Read the model definition and answer for the solid it produces. Units are mm, in the model's axes. A direction names the side the tool comes from. Round coordinates to 2 decimals unless told otherwise and drop trailing zeros. Write each loop counter-clockwise with the first axis right and the second up, starting at its lowest first coordinate (ties: lowest second). Pieces come first, ordered by that corner, then holes. Notation, with made-up numbers: (29, -29) -> (52, -29) arc R18 cw to (52, -11) -> close; hole circle Ø8 at (-29, 62.5). An arc over 180 degrees is marked (long way). Return JSON: item names as keys, results as strings.
from build123d import *

# Parameters (mm, degrees)
F0_W     = 406.4
F0_H     = 508
F1_DEPTH = 3.81
F2_W     = 406.4
F2_H     = 508
F2_W_2   = 398.78
F2_H_2   = 500.38
F3_DEPTH = 38.1


with BuildPart() as f1:
    # F0 (on Front) → F1 (new body)
    with BuildSketch(Plane.XZ):
        with Locations((29.981383, 24.04566)):
            Rectangle(F0_W, F0_H)
    extrude(amount=F1_DEPTH)

    # F2 (on face) → F3 (join)
    with BuildSketch(Plane.XZ.offset(3.81)):
        with Locations((29.981383, 24.04566)):
            Rectangle(F2_W, F2_H)
        with Locations((29.981383, 24.04566)):
            Rectangle(F2_W_2, F2_H_2, mode=Mode.SUBTRACT)
    extrude(amount=F3_DEPTH)


solid = f1.part
Item 1: Section A-A (y = -33) is taken. Give the vertices of the cut face in (x, z), then the cut area to 3 significant figures.
Worked answers:
{"outline": "(-173.22, -229.95) -> (233.18, -229.95) -> (233.18, 278.05) -> (-173.22, 278.05) -> close; hole (-169.41, -226.14) -> (229.37, -226.14) -> (229.37, 274.24) -> (-169.41, 274.24) -> close", "area": "6,910 mm2"}
Item 2: Straight lines are drawn through the part: L1, parallel to X at y = -37, z = -3.5; L2, parallel to Z at x = 191, y = -40; L3, parallel to Y at x = -130, z = 112. For each, find the intervals that lie inside material, in ascending order. Write a range as [from, to].
Worked answers:
{"L1": "x = [-173.22, -169.41], [229.37, 233.18]", "L2": "z = [-229.95, -226.14], [274.24, 278.05]", "L3": "y = [-3.81, 0]"}
Item 3: A flat-ended cylindrical pin translates along its axis: pin 1 (3 mm diameter, centred on x = 139.5, z = -75.5, fed in from -Y). Find the tip coordinate at first contact, or state that the pin passes through.
Worked answers:
{"pin 1": "stops at y = -3.81"}
Item 4: For a pull along X with two mould halves and no side action, classify faces 1 (the flat face through (233.181, -21, 20)), 2 (the flat face through (-169.409, -23, 21)), 3 (the flat face through (27, -23, -226.144)), 4 (the flat face through (27, 0, 28)) as released by +X, released by -X, zero draft, split by the parting line, or undercut.
Worked answers:
{"face 1": "released by +X", "face 2": "undercut", "face 3": "undercut", "face 4": "zero draft"}
Item 5: Section B-B (z = -132) is taken. Give the vertices of the cut face in (x, y), then the cut area to 3 significant figures.
Worked answers:
{"outline": "(-173.22, -41.91) -> (-169.41, -41.91) -> (-169.41, -3.81) -> (229.37, -3.81) -> (229.37, -41.91) -> (233.18, -41.91) -> (233.18, 0) -> (-173.22, 0) -> close", "area": "1,840 mm2"}
Item 6: A tool of negligible diameter and unlimited length cuts with its end or side. For faces 5 (the flat face through (27, -21, -229.954)), 6 (the flat face through (229.371, -23, 21)), from which of +Z, -Z, +X, -X, +Y, -Y can it reach the whole face along a straight path? Write none if from no direction.
Worked answers:
{"face 5": "-Z, +X, -X, +Y, -Y", "face 6": "-Y"}
Item 7: Section C-C (x = -113) is taken. Give the vertices of the cut face in (y, z).
Worked answers:
{"outline": "(-41.91, -229.95) -> (0, -229.95) -> (0, 278.05) -> (-41.91, 278.05) -> (-41.91, 274.24) -> (-3.81, 274.24) -> (-3.81, -226.14) -> (-41.91, -226.14) -> close"}
